Work out the finished part from the listing and answer in its coordinate system (mm). A direction names the side the tool comes from. Coordinates: 2 decimals unless noted, no trailing zeros. Order: outer loops, then holes, each group sorted by start corner. A loop starts at its lowest first (then second) coordinate and runs counter-clockwise, first axis right, second up. Notation, with made-up numbers: M -31,28 L -9,28 A11 ccw -9,46 Z; hole C 66,88 d6. An arc over 180 degrees is marked long. Write item = value, one per line. Start each with the question number.
Q1. Find section B-B on z = -78. Give the vertices of the cut face in (x, y).
Q2. A tool of negligible diameter and unlimited length cuts with its end or side. For faces 4 (the flat face through (-6, 63.5, -2)), 5 (the flat face through (-58, -50.8, 2)), from which of +Z, -Z, +X, -X, +Y, -Y can it reach the whole face along a straight path? Write none if from no direction.
Q3. Find section C-C on x = -69. Give the vertices of the cut face in (y, z).
Q4. Straight lines are drawn through the part: line 1 along X through (y, z) = (47.5, -55); line 2 along Y through (x, z) = (-19, -50). For each, find the intervals that lie inside material, in ascending order.
Q5. Find section A-A on y = 1. Give the vertices of the cut face in (x, z), and give its area (3 significant figures).
Q6. This flat-tipped pin is pushed along its axis until it touches: P1, Ø1.5, axis at y = 14, z = -68, coming from the +X side. Where does it stop, or does it pass through?
Q7. Determine the mould class of faces 1 (the flat face through (-57, -52, -114.3)), 2 (the flat face through (-101.6, 6, 2)), 3 (the flat face through (-114.3, -1, 2)) for opening direction X: released by +X, released by -X, zero draft, split by the parting line, or undercut.
```python
from build123d import *

# Parameters (mm, degrees)
F0_W     = 127
F0_H     = 228.6
F1_DEPTH = 12.7
F4_W     = 127
F4_H     = 228.6
F5_DEPTH = 12.7
F6_W     = 98.14891
F6_H     = 228.6
F7_DEPTH = 12.7


with BuildPart() as f1:
    # F0 (on Right) → F1 (new body)
    with BuildSketch(Plane.YZ):
        Rectangle(F0_W, F0_H)
    extrude(amount=-F1_DEPTH)



with BuildPart() as f5:
    # F4 (on offset) → F5 (new body)
    with BuildSketch(Plane.YZ.offset(-101.6)):
        Rectangle(F4_W, F4_H)
    extrude(amount=-F5_DEPTH)


with BuildPart() as f1_1:
    add(f1.part)

    add(f5.part)  # F7 merges F5
    # F6 (on offset) → F7 (join)
    with BuildSketch(Plane.XZ.offset(50.8)):
        with Locations((-57.461153, 0)):
            Rectangle(F6_W, F6_H)
    extrude(amount=F7_DEPTH)


solid = f1_1.part
```
Findings below:
q1.outline = M -114.3,-63.5 L 0,-63.5 L 0,63.5 L -12.7,63.5 L -12.7,-50.8 L -101.6,-50.8 L -101.6,63.5 L -114.3,63.5 Z
q2.face_4 = +Z, -Z, +X, -X, +Y
q2.face_5 = +Z, -Z, +Y
q3.outline = M -63.5,-114.3 L -50.8,-114.3 L -50.8,114.3 L -63.5,114.3 Z
q4.line_1 = -114.3 to -101.6, -12.7 to 0
q4.line_2 = -63.5 to -50.8
q5.outline = M -114.3,-114.3 L -101.6,-114.3 L -101.6,114.3 L -114.3,114.3 Z; M -12.7,-114.3 L 0,-114.3 L 0,114.3 L -12.7,114.3 Z
q5.area = 5,810 mm^2
q6.P1 = 0
q7.face_1 = zero draft
q7.face_2 = undercut
q7.face_3 = released by -X
